```python
from build123d import *

# Parameters (mm, degrees)
M3_TAPPED_HOLE1_D     = 2.5
M3_TAPPED_HOLE1_DEPTH = 7.5
M3_TAPPED_HOLE1_TIP   = 0.751075774
SKETCH5_W             = 11.224279957
SKETCH5_H             = 5.216918853
SKETCH5_W_2           = 10.939720747
SKETCH5_H_2           = 5.185301163
CUT_EXTRUDE1_DEPTH    = 5
SKETCH6_R             = 1.5
BOSS_EXTRUDE1_DEPTH   = 2
BOSS_EXTRUDE2_DEPTH   = 15


with BuildPart() as part:
    # Sketch1 → Revolve1 (revolve)
    with BuildSketch(Plane.XY):
        Polygon((0, 0), (-16, 0), (-16, 12), (-13, 12), (-13, 14), (-12.25, 14), (-12.25, 25.2), (0, 25.2), align=None)
    revolve(axis=Axis((0, 0, 0), (0, 1, 0)))

    # Sketch2 → Revolve2 (revolve)
    with BuildSketch(Plane.XY):
        Polygon((4, -2.7), (4, -1.25), (3.5, -1.25), (3.5, 0), (8, 0), (8, -10.2), (5.5, -10.2), (5.5, -2.7), align=None)
    revolve(axis=Axis((8, 0, 0), (0, -1, 0)))

    # M3 Tapped Hole1
    with Locations(Plane(origin=(0, -10.2, 0), x_dir=(-1, 0, 0), z_dir=(0, -1, 0))):
        with Locations((-8, 0)):
            Hole(M3_TAPPED_HOLE1_D / 2, depth=M3_TAPPED_HOLE1_DEPTH)
            with Locations((0, 0, -(M3_TAPPED_HOLE1_DEPTH + M3_TAPPED_HOLE1_TIP / 2))):  # 118° drill point
                Cone(0, M3_TAPPED_HOLE1_D / 2, M3_TAPPED_HOLE1_TIP, mode=Mode.SUBTRACT)

    # Sketch5 → Cut-Extrude1 (cut)
    with BuildSketch(Plane.XZ.offset(10.2)):
        with Locations((7.653051139, 4.608459426)):
            Rectangle(SKETCH5_W, SKETCH5_H)
        with Locations((7.795330744, -4.592650582)):
            Rectangle(SKETCH5_W_2, SKETCH5_H_2)
    extrude(amount=-CUT_EXTRUDE1_DEPTH, mode=Mode.SUBTRACT)

    # Sketch6 → Boss-Extrude1 (add)
    with BuildSketch(Plane.XZ):
        with BuildLine():
            Line((-4, -19.5), (-4, 19.5))
            ThreePointArc((-4, 19.5), (0, 23.5), (4, 19.5))
            Line((4, 19.5), (4, -19.5))
            ThreePointArc((4, -19.5), (0, -23.5), (-4, -19.5))
        make_face()
        with Locations((0, -19.5)):
            Circle(SKETCH6_R, mode=Mode.SUBTRACT)
        with Locations((0, 19.5)):
            Circle(SKETCH6_R, mode=Mode.SUBTRACT)
    extrude(amount=-BOSS_EXTRUDE1_DEPTH)

    # Sketch7 → Boss-Extrude2 (add)
    with BuildSketch(Plane(origin=(0, 0, 0), x_dir=(0, 0, -1), z_dir=(1, 0, 0))):
        with BuildLine():
            Line((-2.065333305, 24.81029355), (2.065333305, 24.81029355))
            ThreePointArc((2.065333305, 24.81029355), (2.76544629, 24.110180565), (2.065333305, 23.410067581))
            Line((2.065333305, 23.410067581), (-2.065333305, 23.410067581))
            ThreePointArc((-2.065333305, 23.410067581), (-2.76544629, 24.110180565), (-2.065333305, 24.81029355))
        make_face()
    extrude(amount=-BOSS_EXTRUDE2_DEPTH)


solid = part.part
```
Work out the finished part from the listing and answer in its coordinate system (mm). A direction names the side the tool comes from. Give positions to 0.01 mm unless a question says otherwise; leave off trailing zeros. Order: outer loops, then holes, each group sorted by start corner. A loop starts at its lowest first (then second) coordinate and runs counter-clockwise, first axis right, second up.
1. For faces 1 (the flat face through (5, -1.25, 3)), 2 (the flat face through (-4, 1, 17)), 3 (the flat face through (8, -8, -2)), 4 (the flat face through (8, -8, 2)), 5 (the cylindrical face through (0.1, 1, -23.5)), determine the directions among +Z, -Z, +X, -X, +Y, -Y from which every point of the face is accessible in a straight line to the end or side of a thin tool.
Result sheet:
face 1: -Y
face 2: +Z, -X, +Y, -Y
face 3: -Z, +X, -X, -Y
face 4: +Z, +X, -X, -Y
face 5: -Z, +Y, -Y
2. Section D-D, the plane x = -11 is taken. Determine the outline of the cut face in (y, z).
Result sheet:
outline: (0, -11.62) - (12, -11.62) - (12, -6.93) - (14, -6.93) - (14, -5.39) - (25.2, -5.39) - (25.2, 5.39) - (14, 5.39) - (14, 6.93) - (12, 6.93) - (12, 11.62) - (0, 11.62) - close
3. Each of these flat-tipped pins is pushed along its axis until it touches: P1, Ø1.6, axis at y = 1, z = 17.5, coming from the -X side; P2, Ø1, axis at x = -6.5, y = 5.5, coming from the +Z side; P3, Ø4, axis at x = 0, z = -19.5, coming from the +Y side; P4, Ø12, axis at y = -3, z = 4, coming from the -X side. Where does it stop, or does it pass through?
Result sheet:
P1: stops at x = -4
P2: stops at z = 14.83
P3: stops at y = 2
P4: stops at x = -16
4. The mould has two halves that part along X. Classify faces 6 (the flat face through (6, -2.7, 2)), 7 (the flat face through (4, 1, 18)), 8 (the cylindrical face through (3.708, -0.616, -1.352)), 9 (the cylindrical face through (6.75, -6.4, -0.05)): released by +X, released by -X, zero draft, split by the parting line, or undercut.
Result sheet:
face 6: zero draft
face 7: released by +X
face 8: split by the parting line
face 9: undercut
5. Section B-B, the plane x = 0 is taken. Determine the outline of the cut face in (y, z), and give its area (3 significant figures).
Result sheet:
outline: (0, -23.5) - (2, -23.5) - (2, -21) - (0, -21) - close; (0, -18) - (2, -18) - (2, -16) - (12, -16) - (12, -13) - (14, -13) - (14, -12.25) - (25.2, -12.25) - (25.2, 12.25) - (14, 12.25) - (14, 13) - (12, 13) - (12, 16) - (2, 16) - (2, 18) - (0, 18) - close; (0, 21) - (2, 21) - (2, 23.5) - (0, 23.5) - close
area: 728 mm2
6. Straight lines are drawn through the part: L1, parallel to Z at x = 0, y = 0.6; L2, parallel to Y at x = 2.5, z = 6.5; L3, parallel to X at y = 1, z = -4. For each, find the intervals that lie inside material, in ascending order.
Result sheet:
L1: z = -23.5 to -21, -18 to 18, 21 to 23.5
L2: y = 0 to 25.2
L3: x = -15.49 to 15.49
7. Section A-A, the plane y = -8 is taken. Determine the outline of the cut face in (x, z).
Result sheet:
outline: (6.5, -2) - (9.5, -2) arc R2.5 ccw to (9.5, 2) - (6.5, 2) arc R2.5 ccw to start; hole circle Ø2.5 at (8, 0)
8. Section C-C, the plane z = -10 is taken. Determine the outline of the cut face in (x, y).
Result sheet:
outline: (-12.49, 0) - (12.49, 0) - (12.49, 12) - (8.31, 12) - (8.31, 14) - (7.08, 14) - (7.08, 25.2) - (-7.08, 25.2) - (-7.08, 14) - (-8.31, 14) - (-8.31, 12) - (-12.49, 12) - close
